The drawing under review shows one solid part. Ordinate dimensions are in mm from its lowest x, y, z. A direction names the side the tool comes from. Coordinates: 2 decimals unless noted, no trailing zeros. Order: outer loops, then holes, each group sorted by start corner. A loop starts at its lowest first (then second) coordinate and runs counter-clockwise, first axis right, second up. Notation, with made-up numbers: M 0.5,-11 L 14.5,-11 A24 ccw 14.5,5 Z; hole C -27,8 d7. An arc over 180 degrees is marked long. Answer as a JSON object with one key per item and string values.
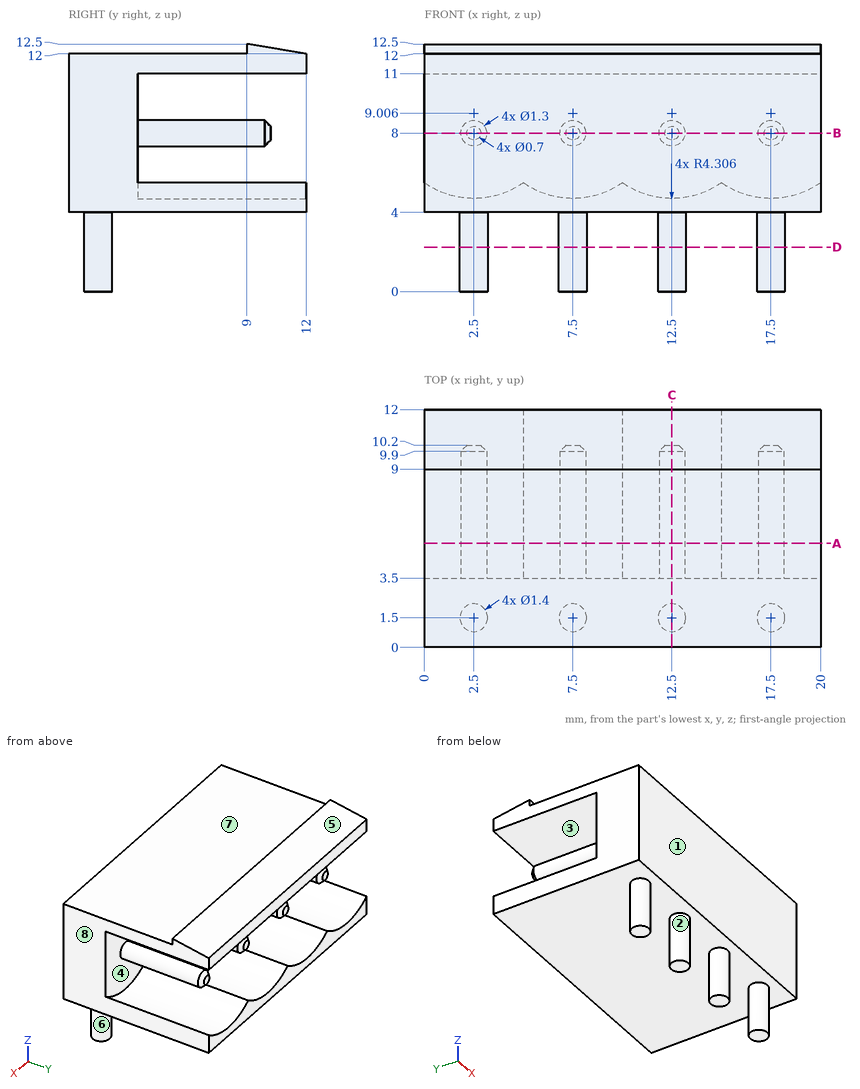
1) Add section B-B (z = 8). State the section outline as (x, y) points.
Taken from the geometry:
{"outline": "M 0,0 L 20,0 L 20,3.5 L 18.15,3.5 L 18.15,9.9 L 17.85,10.2 L 17.15,10.2 L 16.85,9.9 L 16.85,3.5 L 13.15,3.5 L 13.15,9.9 L 12.85,10.2 L 12.15,10.2 L 11.85,9.9 L 11.85,3.5 L 8.15,3.5 L 8.15,9.9 L 7.85,10.2 L 7.15,10.2 L 6.85,9.9 L 6.85,3.5 L 3.15,3.5 L 3.15,9.9 L 2.85,10.2 L 2.15,10.2 L 1.85,9.9 L 1.85,3.5 L 0,3.5 Z"}
2) Add section C-C (x = 12.5). State the section outline as (y, z) points.
Taken from the geometry:
{"outline": "M 0,4 L 0.8,4 L 0.8,0 L 2.2,0 L 2.2,4 L 12,4 L 12,4.7 L 3.5,4.7 L 3.5,7.35 L 9.9,7.35 L 10.2,7.65 L 10.2,8.35 L 9.9,8.65 L 3.5,8.65 L 3.5,11 L 12,11 L 12,12 L 9,12.5 L 9,12 L 0,12 Z"}
3) Mouldability with a two-part tool opening along X and no side actions: class the marked faces 6, 7 and 8 as released by +X, released by -X, zero draft, split by the parting line, or undercut.
Taken from the geometry:
{"face 6": "undercut", "face 7": "zero draft", "face 8": "released by +X"}
4) To check wall thickness, follow L1, parallel to X at y = 5.5, z = 7.5 (1 decimal); L2, parallel to Z at x = 9.75, y = 1.25; L3, parallel to Y at x = 11.5, z = 10. State the ranges of each line that lie inside material, in increasing order.
Taken from the geometry:
{"L1": "x = 2.1 to 2.9, 7.1 to 7.9, 12.1 to 12.9, 17.1 to 17.9", "L2": "z = 4 to 12", "L3": "y = 0 to 3.5"}
5) Tool access review of the marked faces 1, 2, 3, 4 and 5: name each direction out of +Z, -Z, +X, -X, +Y, -Y from which nothing blocks a thin tool from reaching the whole face with its end or side.
Taken from the geometry:
{"face 1": "+Z, -Z, +X, -X, -Y", "face 2": "-Z", "face 3": "+X, -X, +Y", "face 4": "+Y", "face 5": "+Z, +X, -X, +Y"}
6) Add section D-D (z = 2.25). State the section outline as (x, y) points.
Taken from the geometry:
{"outline": "C 2.5,1.5 d1.4; C 7.5,1.5 d1.4; C 12.5,1.5 d1.4; C 17.5,1.5 d1.4"}
7) Add section A-A (y = 5.25). State the section outline as (x, z) points.
Taken from the geometry:
{"outline": "M 0,4 L 20,4 L 20,5.5 A4.31 cw 15,5.5 A4.31 cw 10,5.5 A4.31 cw 5,5.5 A4.31 cw 0,5.5 Z; M 0,11 L 20,11 L 20,12 L 0,12 Z; C 2.5,8 d1.3; C 7.5,8 d1.3; C 12.5,8 d1.3; C 17.5,8 d1.3"}
8) Insertion check: pin 1 Ø3 at (x, z) = (18, 7.5) entering from -Y; pin 2 Ø1 at (x, y) = (4, 3.5) entering from -Z; pin 3 Ø2 at (x, z) = (17, 8) entering from +Y; pin 4 Ø3 at (x, z) = (9.5, 7.5) entering from +Y. Each pin has a flat end and moves straight along its axis. Give the tip position at first contact, or say it passes through.
Taken from the geometry:
{"pin 1": "stops at y = 0", "pin 2": "stops at z = 4", "pin 3": "stops at y = 10.2", "pin 4": "stops at y = 9.99"}
